Build history of the part. All positions in model axes, mm. A direction names the side the tool comes from. Coordinates: 2 decimals unless noted, no trailing zeros. Loops run counter-clockwise (first coordinate to the right, second up) from the corner with the lowest first, then second, coordinate; pieces in that order, holes last.
(1) Slice it at D-D (z = 1). Give the cut face in (x, y), and give its area (3 significant figures).
(2) Two-plate mould, pull along X, no slides. Class faces 1 (the face through (-14, 30, 4)), 2 (the face through (30, -14, 4)), 3 (the face through (22.996, 21.086, -2.535)), 4 (the face through (14, 30, 4)): pulls with the +X half, pulls with the -X half, needs draft (parallel to the pull), parting line crosses it, or undercut.
(3) Tool access for faces 5 (the face through (-14, -30, 4)), 6 (the face through (0, 30, 4)), 7 (the face through (-30, 14, 4)), 8 (the face through (-3.233, -1.341, -3.944)): list every direction of +Z, -Z, +X, -X, +Y, -Y with a clear straight run to the whole face (end or side of a thin tool).
(4) Slice it at C-C (z = 5.25). Give the cut face in (x, y).
(5) Flat gauge pins, fed straight in: P1, Ø2, axis at x = 25.5, y = -16, coming from the +Z side; P2, Ø1, axis at y = -19, z = -1, coming from the +X side; P3, Ø2, axis at y = 29.5, z = 5, coming from the +X side. Where does each tip first touch, or does it go through?
(6) Wall check: L1, parallel to Y at x = 0, z = 1.5; L2, parallel to Y at x = 0, z = -2.95; L3, parallel to Y at x = -33, z = 4.5. Give the ranges that are in metal, low to high.
(7) Slice it at A-A (z = -2.75). Give the cut face in (x, y), and give its area (3 significant figures).
(8) Slice it at B-B (x = 0). Give the cut face in (y, z), and give its area (4 significant figures).
from build123d import *

# Parameters (mm, degrees)
SKETCH_1_R          = 36.5
EXTRUDE_1_DEPTH     = 6.5
CUT_EXTRUDE_START   = -4
CUT_EXTRUDE_2_DEPTH = 4
CUT_EXTRUDE_3_DEPTH = 4
SKETCH_6_R          = 1.5
CUT_EXTRUDE_5_DEPTH = 53.026435588
EXTRUDE_START       = 5
SKETCH_7_R          = 36.5
SKETCH_7_R_2        = 1.5
EXTRUDE_2_DEPTH     = 5
SKETCH_8_R          = 31.2
CUT_EXTRUDE_6_DEPTH = 5
SKETCH_9_R          = 3.5
EXTRUDE_3_DEPTH     = 8


with BuildPart() as part:
    # 草图1 → 凸台-拉伸1 (new body)
    with BuildSketch(Plane.XY):
        with Locations(Location((0, 0, 0), (0, 0, 180))):
            Circle(SKETCH_1_R)
    extrude(amount=EXTRUDE_1_DEPTH)

    # 草图3 → 切除-拉伸2 (cut)
    with BuildSketch(Plane.XY.offset(6.5).offset(CUT_EXTRUDE_START)):
        with BuildLine():
            Line((14, 33.708307581), (14, 26.532998323))
            ThreePointArc((14, 26.532998323), (21.213203436, 21.213203436), (26.532998323, 14))
            Line((26.532998323, 14), (33.708307581, 14))
            ThreePointArc((33.708307581, 14), (25.809397513, 25.809397513), (14, 33.708307581))
        make_face()
        with BuildLine():
            ThreePointArc((26.532998323, -14), (21.213203436, -21.213203436), (14, -26.532998323))
            Line((14, -26.532998323), (14, -33.708307581))
            ThreePointArc((14, -33.708307581), (25.809397513, -25.809397513), (33.708307581, -14))
            Line((33.708307581, -14), (26.532998323, -14))
        make_face()
        with BuildLine():
            Line((-14, -33.708307581), (-14, -26.532998323))
            ThreePointArc((-14, -26.532998323), (-21.213203436, -21.213203436), (-26.532998323, -14))
            Line((-26.532998323, -14), (-33.708307581, -14))
            ThreePointArc((-33.708307581, -14), (-25.809397513, -25.809397513), (-14, -33.708307581))
        make_face()
        with BuildLine():
            Line((-33.708307581, 14), (-26.532998323, 14))
            ThreePointArc((-26.532998323, 14), (-21.213203436, 21.213203436), (-14, 26.532998323))
            Line((-14, 26.532998323), (-14, 33.708307581))
            ThreePointArc((-14, 33.708307581), (-25.809397513, 25.809397513), (-33.708307581, 14))
        make_face()
    extrude(amount=CUT_EXTRUDE_2_DEPTH, mode=Mode.SUBTRACT)

    # 草图4 → 切除-拉伸3 (cut)
    with BuildSketch(Plane.XY.offset(6.5).offset(CUT_EXTRUDE_START)):
        with BuildLine():
            ThreePointArc((26.532998323, -14), (29.120353275, -7.211450974), (30, 0))
            ThreePointArc((30, 0), (29.120353275, 7.211450974), (26.532998323, 14))
            ThreePointArc((26.532998323, 14), (21.213203436, 21.213203436), (14, 26.532998323))
            ThreePointArc((14, 26.532998323), (0, 30), (-14, 26.532998323))
            ThreePointArc((-14, 26.532998323), (-21.213203436, 21.213203436), (-26.532998323, 14))
            ThreePointArc((-26.532998323, 14), (-30, 0), (-26.532998323, -14))
            ThreePointArc((-26.532998323, -14), (-21.213203436, -21.213203436), (-14, -26.532998323))
            ThreePointArc((-14, -26.532998323), (0, -30), (14, -26.532998323))
            ThreePointArc((14, -26.532998323), (21.213203436, -21.213203436), (26.532998323, -14))
        make_face()
    extrude(amount=CUT_EXTRUDE_3_DEPTH, mode=Mode.SUBTRACT)

    # 草图6 → 切除-拉伸5 (cut, through all)
    with BuildSketch(Plane(origin=(0, 0, 0), x_dir=(-1, 0, 0), z_dir=(0, 0, -1))):
        with Locations((32.9, 0)):
            Circle(SKETCH_6_R)
        with Locations((0, -32.9)):
            Circle(SKETCH_6_R)
        with Locations((0, 32.9)):
            Circle(SKETCH_6_R)
        with Locations((-32.9, 0)):
            Circle(SKETCH_6_R)
    extrude(amount=-CUT_EXTRUDE_5_DEPTH, mode=Mode.SUBTRACT)

    # 草图7 → 凸台-拉伸2 (add)
    with BuildSketch(Plane(origin=(0, 0, 0), x_dir=(-1, 0, 0), z_dir=(0, 0, -1)).offset(EXTRUDE_START)):
        Circle(SKETCH_7_R)
        with Locations((0, -32.9)):
            Circle(SKETCH_7_R_2, mode=Mode.SUBTRACT)
        with Locations((-32.9, 0)):
            Circle(SKETCH_7_R_2, mode=Mode.SUBTRACT)
        with Locations((0, 32.9)):
            Circle(SKETCH_7_R_2, mode=Mode.SUBTRACT)
        with Locations((32.9, 0)):
            Circle(SKETCH_7_R_2, mode=Mode.SUBTRACT)
    extrude(amount=-EXTRUDE_2_DEPTH)

    # 草图8 → 切除-拉伸6 (cut)
    with BuildSketch(Plane(origin=(0, 0, -5), x_dir=(-1, 0, 0), z_dir=(0, 0, -1))):
        Circle(SKETCH_8_R)
    extrude(amount=-CUT_EXTRUDE_6_DEPTH, mode=Mode.SUBTRACT)

    # 草图9 → 凸台-拉伸3 (add)
    with BuildSketch(Plane(origin=(0, 0, 0), x_dir=(-1, 0, 0), z_dir=(0, 0, -1))):
        Circle(SKETCH_9_R)
    extrude(amount=EXTRUDE_3_DEPTH)


solid = part.part
Response values:
1. outline: circle Ø73 at (0, 0); hole circle Ø3 at (-32.9, 0); hole circle Ø3 at (0, -32.9); hole circle Ø3 at (0, 32.9); hole circle Ø3 at (32.9, 0)
1. area: 4,160 mm2
2. face 1: pulls with the -X half
2. face 2: needs draft
2. face 3: undercut
2. face 4: pulls with the +X half
3. face 5: +Z, -X, +Y, -Y
3. face 6: +Z
3. face 7: +Z, +X, -X, +Y
3. face 8: -Z
4. outline: (-33.71, -14) - (-26.53, -14) arc R30 cw to (-26.53, 14) - (-33.71, 14) arc R36.5 ccw to start; (-14, -33.71) arc R36.5 ccw to (14, -33.71) - (14, -26.53) arc R30 cw to (-14, -26.53) - close; (-14, 26.53) arc R30 cw to (14, 26.53) - (14, 33.71) arc R36.5 ccw to (-14, 33.71) - close; (26.53, -14) - (33.71, -14) arc R36.5 ccw to (33.71, 14) - (26.53, 14) arc R30 cw to start; hole circle Ø3 at (-32.9, 0); hole circle Ø3 at (0, -32.9); hole circle Ø3 at (0, 32.9); hole circle Ø3 at (32.9, 0)
5. P1: stops at z = 2.5
5. P2: stops at x = 31.46
5. P3: stops at x = 14
6. L1: y = -36.5 to -34.4, -31.4 to 31.4, 34.4 to 36.5
6. L2: y = -36.5 to -34.4, -31.4 to -31.2, -3.5 to 3.5, 31.2 to 31.4, 34.4 to 36.5
6. L3: y = -14 to -1.5, 1.5 to 14
7. outline: circle Ø73 at (0, 0); circle Ø7 at (0, 0); hole circle Ø3 at (-32.9, 0); hole circle Ø62.4 at (0, 0); hole circle Ø3 at (0, -32.9); hole circle Ø3 at (0, 32.9); hole circle Ø3 at (32.9, 0)
7. area: 1,140 mm2
8. outline: (-36.5, -5) - (-34.4, -5) - (-34.4, 6.5) - (-36.5, 6.5) - close; (-31.4, -5) - (-31.2, -5) - (-31.2, 0) - (-3.5, 0) - (-3.5, -8) - (3.5, -8) - (3.5, 0) - (31.2, 0) - (31.2, -5) - (31.4, -5) - (31.4, 6.5) - (30, 6.5) - (30, 2.5) - (-30, 2.5) - (-30, 6.5) - (-31.4, 6.5) - close; (34.4, -5) - (36.5, -5) - (36.5, 6.5) - (34.4, 6.5) - close
8. area: 274.5 mm2
